Can you work these out from the model? Positions are in its coordinate system, mm. Face numbers are marked on the shaded views. A direction names the side the tool comes from. Give positions to 0.01 mm unless a question says otherwise; leave off trailing zeros. Loops run counter-clockwise (first coordinate to the right, second up) from the corner with the lowest first, then second, coordinate; pieces in that order, holes last. Notation, with made-up numbers: (89.25, 16.5) -> (111.25, 16.5) arc R20 ccw to (111.25, 48.5) -> close; hole circle Ø7 at (25, 11). An arc over 180 degrees is marked (long way). Return JSON: item names as keys, results as strings. Group by question number.
Q1. I need wall thicknesses on line 1 along Y through (x, z) = (24, -41); line 2 along Z through (x, y) = (14.75, 6.35); line 3 along Y through (x, z) = (10.25, -88.9). Which ranges of each line are inside material? Lowest first, please. Write a range as [from, to].
Q2. Thinking about a two-plate mould opening in Z: for the marked faces 4, 5 and 6, which applies, pulls with the +Z half, pulls with the -Z half, needs draft (parallel to the pull), parting line crosses it, or undercut?
Q3. Suppose I cut it at C-C, the plane y = 6.35. Please give me the cut outline in (x, z).
Q4. Suppose I cut it at B-B, the plane z = -88.9. Please give me the cut outline in (x, y) (3 decimals).
Q5. Will these pins go through, and if not, where does the flat tip stop? pin 1 (8 mm diameter, centred on x = 6.5, y = 88.5, fed in from +Z); pin 2 (4 mm diameter, centred on y = 6.35, z = -88.9, fed in from -X).
Q6. Which directions (+Z, -Z, +X, -X, +Y, -Y) give clear straight access to the entire face, cutting with the end or side of a thin tool? Please do the marked faces 1, 2 and 3.
Q7. Suppose I cut it at A-A, the plane x = 16.25. Count the separate pieces of the cut face and the enclosed holes in it, and give its area (3 significant figures).
Autodesk Inventor part; units mm, degrees
ref_plane "YZ Plane" through (0, 0, 0) normal (1, 0, 0) x (0, 1, 0)
ref_plane "XZ Plane" through (0, 0, 0) normal (0, 1, 0) x (-1, 0, 0)
ref_plane "XY Plane" through (0, 0, 0) normal (0, 0, 1) x (1, 0, 0)
sketch "Sketch1" plane through (0, 0, 0) normal (1, 0, 0) x (0, 1, 0)
  line L0 (0, 0) -> (101.6, 0)
  line L1 (101.6, 0) -> (101.6, -101.6)
  line L2 (101.6, -101.6) -> (0, -101.6)
  line L3 (0, -101.6) -> (0, 0)
  dimension "d0" = 101.6
  dimension "d1" = 101.6
extrude "Extrusion1" add sketch "Sketch1" along normal blind 25.4
sketch "Sketch2" plane through (25.4, 0, 0) normal (1, 0, 0) x (0, 0, -1)
  line L0 (0, 101.6) -> (0, 0)
  line L1 (0, 0) -> (12.7, 0)
  line L2 (12.7, 0) -> (12.7, 6.35)
  line L3 (12.7, 6.35) -> (0, 6.35)
  line L4 (0, 6.35) -> (0, 0)
  line L5 (101.6, 0) -> (101.6, 101.6)
  line L6 (101.6, 0) -> (88.9, 0)
  line L7 (88.9, 0) -> (88.9, 6.35)
  line L8 (88.9, 6.35) -> (101.6, 6.35)
  line L9 (101.6, 6.35) -> (101.6, 0)
  line L10 (101.6, 101.6) -> (0, 101.6)
  line L11 (50.8, 101.6) -> (50.8, 76.2)
  line L12 (25.273, 58.7121) -> (76.327, 58.7121)
  line L13 (76.327, 58.7121) -> (76.327, 93.6879)
  line L14 (76.327, 93.6879) -> (25.273, 93.6879)
  line L15 (25.273, 93.6879) -> (25.273, 58.7121)
  line L16 (25.273, 58.7121) -> (76.327, 93.6879) construction
  line L17 (76.327, 58.7121) -> (25.273, 93.6879) construction
  line L18 (74.9076, 71.12) -> (101.6, 71.12)
  line L19 (101.6, 71.12) -> (101.6, 81.28)
  line L20 (101.6, 81.28) -> (74.9076, 81.28)
  line L21 (74.9076, 81.28) -> (74.9076, 71.12)
  line L22 (74.9076, 71.12) -> (101.6, 81.28) construction
  line L23 (101.6, 71.12) -> (74.9076, 81.28) construction
  line L24 (25.273, 93.6879) -> (25.273, 83.5279)
  line L25 (25.273, 58.7121) -> (25.273, 70.1421)
  line L26 (25.273, 70.1421) -> (0, 81.28)
  line L27 (25.273, 83.5279) -> (0, 95.6039)
  line L28 (0, 81.28) -> (0, 95.6039)
  line L29 (25.273, 83.5279) -> (25.273, 70.1421)
  point P0 (88.2538, 76.2)
  point P1 (76.327, 81.28)
  point P2 (76.327, 71.12)
  dimension "d4" = 12.7
  dimension "d5" = 6.35
  dimension "d6" = 12.7
  dimension "d7" = 6.35
  dimension "d8" = 25.4
  dimension "d9" = 51.054
  dimension "d10" = 34.9758
  dimension "d20" = 10.16
  dimension "d21" = 10.16
  dimension "d22" = 11.43
extrude "Extrusion2" cut sketch "Sketch2" against normal blind 25.4 contours L27 L15 L26 L0 | L15 L14 L13 L20 L21 L18 L12 | L5 L18 L13 L20 | L13 L18 L21 L20
hole "Hole1" at (25.4, 6.35, -88.9) at (25.4, 6.35, -12.7) direction (-1, 0, 0) diameter 4.9784 end through all
sketch "Sketch5" plane through (25.4, 0, 0) normal (1, 0, 0) x (0, 0, -1)
  line L0 (0, 101.6) -> (0, 95.6039)
  line L1 (25.273, 58.7121) -> (76.327, 58.7121)
  line L2 (0, 101.6) -> (25.273, 101.6)
  line L3 (25.273, 101.6) -> (25.273, 58.7121)
  line L4 (25.273, 58.7121) -> (0, 58.7121)
  line L5 (0, 58.7121) -> (0, 101.6)
  line L6 (101.6, 81.28) -> (101.6, 101.6)
  line L7 (76.327, 58.7121) -> (101.6, 58.7121)
  line L8 (101.6, 58.7121) -> (101.6, 101.6)
  line L9 (101.6, 101.6) -> (76.327, 101.6)
  line L10 (76.327, 101.6) -> (76.327, 58.7121)
  point P0 (0, 0)
extrude "Extrusion4" add sketch "Sketch5" against normal blind 3.175
sketch "Sketch6" plane through (25.4, 0, 0) normal (1, 0, 0) x (0, 0, -1)
  line L0 (76.327, 93.6879) -> (25.273, 93.6879)
  line L1 (50.8, 93.6879) -> (43.7642, 93.6879)
  line L2 (43.7642, 93.6879) -> (43.7642, 97.6503)
  line L3 (101.6, 101.6) -> (0, 101.6)
  line L4 (40.4622, 100.9523) -> (47.0662, 100.9523)
  line L5 (47.0662, 100.9523) -> (47.0662, 94.3483)
  line L6 (47.0662, 94.3483) -> (40.4622, 94.3483)
  line L7 (40.4622, 94.3483) -> (40.4622, 100.9523)
  line L8 (40.4622, 100.9523) -> (47.0662, 94.3483) construction
  line L9 (47.0662, 100.9523) -> (40.4622, 94.3483) construction
  point P0 (0, 0)
  dimension "d30" = 7.0358
  dimension "d31" = 3.9624
  dimension "d32" = 6.604
  dimension "d33" = 6.604
extrude "Extrusion5" cut sketch "Sketch6" against normal blind 25.4
sketch "Sketch7" plane through (0, 101.6, 0) normal (0, 1, 0) x (1, 0, 0)
  line L0 (25.4, 40.4622) -> (0, 40.4622)
  line L1 (25.4, 47.0662) -> (0, 47.0662)
  line L2 (0, 47.0662) -> (0, 43.7642)
  line L3 (0, 101.6) -> (0, 0)
  line L4 (0, 43.7642) -> (3.94, 43.7642)
  dimension "d36" = 3.302
  dimension "d37" = 3.94
hole "Hole2" at (3.94, 101.6, -43.7642) direction (0, -1, 0) diameter 4.318 depth 6.35 tip angle 118
sketch "Sketch8" plane through (25.4, 94.3483, -40.4622) normal (0, 1, 0) x (1, 0, 0)
  point P0 (-25.4, -40.4622)
  point P1 (-21.46, 3.302)
hole "Hole3" at (3.94, 94.3483, -43.7642) direction (0, -1, 0) diameter 2.6416 depth 10.9728 tip angle 118
sketch "Sketch9" plane through (25.4, 0, 0) normal (1, 0, 0) x (0, 0, -1)
  line L0 (25.273, 93.6879) -> (76.327, 93.6879)
  line L1 (25.273, 93.6879) -> (25.273, 92.1004)
  line L2 (25.273, 58.7121) -> (25.273, 93.6879)
  circle A0 centre (25.273, 92.1004) radius 1.5875
  line L3 (25.273, 58.7121) -> (25.273, 60.2996)
  line L4 (76.327, 93.6879) -> (76.327, 92.1004)
  line L5 (76.327, 93.6879) -> (76.327, 58.7121)
  line L6 (25.273, 58.7121) -> (76.327, 58.7121)
  line L7 (76.327, 58.7121) -> (76.327, 60.2996)
  line L8 (40.4622, 100.9523) -> (40.4622, 94.3483)
  line L9 (40.4622, 94.3483) -> (40.4622, 95.9358)
  line L10 (40.4622, 100.9523) -> (40.4622, 99.3648)
  line L11 (47.0662, 100.9523) -> (47.0662, 99.3648)
  line L12 (47.0662, 94.3483) -> (47.0662, 100.9523)
  line L13 (47.0662, 94.3483) -> (47.0662, 95.9358)
  circle A1 centre (25.273, 60.2996) radius 1.5875
  circle A2 centre (76.327, 60.2996) radius 1.5875
  circle A3 centre (76.327, 92.1004) radius 1.5875
  circle A4 centre (47.0662, 99.3648) radius 1.5875
  circle A5 centre (47.0662, 95.9358) radius 1.5875
  circle A6 centre (40.4622, 95.9358) radius 1.5875
  circle A7 centre (40.4622, 99.3648) radius 1.5875
  point P0 (0, 0)
  point P1 (76.327, 90.5129)
  point P2 (76.327, 61.8871)
  dimension "d52" = 1.5875
  dimension "d53" = 3.175
  dimension "d54" = 1.5875
  dimension "d55" = 1.5875
  dimension "d56" = 1.5875
  dimension "d57" = 1.5875
  dimension "d58" = 1.5875
  dimension "d59" = 1.5875
  dimension "d60" = 1.5875
  dimension "d61" = 3.175
  dimension "d62" = 3.175
  dimension "d63" = 3.175
  dimension "d64" = 3.175
  dimension "d65" = 3.175
  dimension "d66" = 3.175
  dimension "d67" = 3.175
extrude "Extrusion6" cut sketch "Sketch9" against normal blind 25.4 contours A0 L2 L1 | L1 L2 A0 | A3 L5 L4 | A1 L2 | L2 A1 | A2 L5 | A7 L8 | A6 L8 | L8 A6 | L8 A7 | A4 L12 L11 | A5 L12 | L12 A5 | L11 L12 A4 picked at (76.6743, 93.0931) picked at (76.6743, 59.3069)
properties part number "Al thermal core-r2"
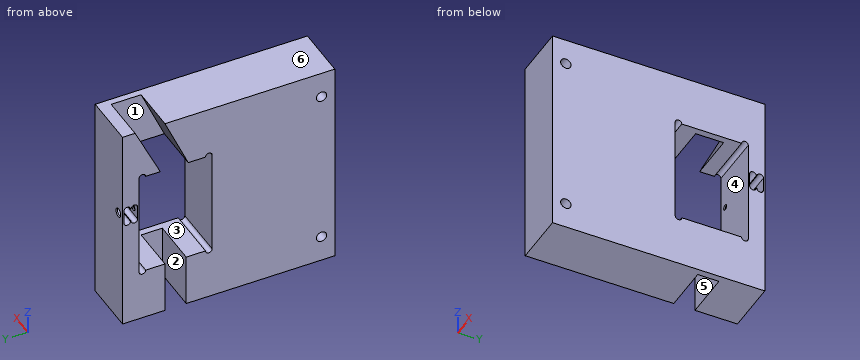
Ans:
{
 "1": {"line 1": "y = [0, 58.71], [93.69, 94.35], [100.95, 101.6]", "line 2": "z = [-101.6, -91.39], [-86.41, -15.19], [-10.21, 0]", "line 3": "y = [0, 3.86], [8.84, 71.12], [81.28, 101.6]"},
 "2": {"face 4": "undercut", "face 5": "needs draft", "face 6": "pulls with the +Z half"},
 "3": {"outline": "(0, -101.6) -> (25.4, -101.6) -> (25.4, -91.39) -> (0, -91.39) -> close; (0, -86.41) -> (25.4, -86.41) -> (25.4, -15.19) -> (0, -15.19) -> close; (0, -10.21) -> (25.4, -10.21) -> (25.4, 0) -> (0, 0) -> close"},
 "4": {"outline": "(0, 0) -> (25.4, 0) -> (25.4, 3.861) -> (0, 3.861) -> close; (0, 8.839) -> (25.4, 8.839) -> (25.4, 101.6) -> (0, 101.6) -> (0, 81.28) -> (22.225, 81.28) -> (22.225, 71.12) -> (0, 71.12) -> close"},
 "5": {"pin 1": "stops at z = -6.5", "pin 2": "passes through"},
 "6": {"face 1": "-X", "face 2": "-Z, -X", "face 3": "+X, -X"},
 "7": {"separate pieces": "2", "enclosed holes": "3", "area": "7,820 mm^2"}
}
